```python
from build123d import *

# Parameters (mm, degrees)
BASE_FLANGE1_DEPTH  = 50.8
SKETCH3_R           = 2.7051
TAB1_DEPTH          = 6.35
SKETCH3_2_R         = 2.7051
CUT_EXTRUDE1_DEPTH  = 12.7
SKETCH4_R           = 3.5687
CUT_EXTRUDE2_DEPTH  = 12.7
FILLET1_R           = 6.35
UNFOLD1_START       = 6.35
UNFOLD1_OUTLINE_W   = 50.8
UNFOLD1_OUTLINE_H   = 14.961835013
UNFOLD1_DEPTH       = 95.25
UNFOLD1_2_OUTLINE_R = 2.7051
UNFOLD1_2_DEPTH     = 6.35
FOLD1_START         = -1.304798
FOLD1_DEPTH         = 92.466633013
FOLD1_START_2       = -6.35
FOLD1_2_OUTLINE_R   = 2.7051
FOLD1_2_DEPTH       = 0.034797996
FOLD1_START_3       = -12.7
FOLD1_3_OUTLINE_R   = 2.7051
FOLD1_3_DEPTH       = 12.7
FOLD1_4_DEPTH       = 50.8


with BuildPart() as part:
    # Base-Flange1: sheet metal written as solids
    # Sketch1 → Base-Flange1 (new body)
    with BuildSketch(Plane(origin=(0, 0, 0), x_dir=(0, 0, -1), z_dir=(1, 0, 0))):
        with BuildLine():
            Line((0, 101.6), (0, 12.7))
            ThreePointArc((0, 12.7), (3.719743879, 3.719743879), (12.7, 0))
            Line((12.7, 0), (50.8, 0))
            Line((50.8, 0), (50.8, 6.35))
            Line((50.8, 6.35), (12.7, 6.35))
            ThreePointArc((12.7, 6.35), (8.209871939, 8.209871939), (6.35, 12.7))
            Line((6.35, 12.7), (6.35, 101.6))
            Line((6.35, 101.6), (0, 101.6))
        make_face()
    extrude(amount=BASE_FLANGE1_DEPTH)

    # Tab1: sheet metal written as solids
    # Sketch3 → Tab1 (add)
    with BuildSketch(Plane(origin=(0, 0, -6.35), x_dir=(-1, 0, 0), z_dir=(0, 0, -1))):
        with Locations((-34.925, 23.114)):
            Circle(SKETCH3_R)
        with Locations((-34.925, 88.9)):
            Circle(SKETCH3_R)
        with Locations((-15.875, 38.608)):
            Circle(SKETCH3_R)
        with Locations((-15.875, 78.486)):
            Circle(SKETCH3_R)
    extrude(amount=-TAB1_DEPTH)

    # Sketch3<2> → Cut-Extrude1 (cut)
    with BuildSketch(Plane(origin=(0, 0, -6.35), x_dir=(-1, 0, 0), z_dir=(0, 0, -1))):
        with Locations(Location((-34.925, 23.114, 0), (0, 0, 90))):
            Circle(SKETCH3_2_R)
        with Locations(Location((-34.925, 88.9, 0), (0, 0, 90))):
            Circle(SKETCH3_2_R)
        with Locations(Location((-15.875, 38.608, 0), (0, 0, 90))):
            Circle(SKETCH3_2_R)
        with Locations(Location((-15.875, 78.486, 0), (0, 0, 90))):
            Circle(SKETCH3_2_R)
    extrude(amount=-CUT_EXTRUDE1_DEPTH, mode=Mode.SUBTRACT)

    # Sketch4 → Cut-Extrude2 (cut)
    with BuildSketch(Plane(origin=(0, 6.35, 0), x_dir=(-1, 0, 0), z_dir=(0, 1, 0))):
        with Locations(Location((-41.275, -19.05, 0), (0, 0, 90))):
            Circle(SKETCH4_R)
        with Locations(Location((-9.525, -41.275, 0), (0, 0, 90))):
            Circle(SKETCH4_R)
    extrude(amount=-CUT_EXTRUDE2_DEPTH, mode=Mode.SUBTRACT)

    # Fillet1
    fillet1_edges = [part.edges().sort_by_distance(p)[0] for p in [
        (50.8, 101.6, -3.175),
        (0, 101.6, -3.175),
        (50.8, 3.175, -50.8),
        (0, 3.175, -50.8),
    ]]
    fillet(fillet1_edges, radius=FILLET1_R)

    # Unfold1: read off the stored shape, not the designer's step
    # Unfold1 outline → Unfold1 (cut)
    with BuildSketch(Plane(origin=(0, 0, 0), x_dir=(1, 0, 0), z_dir=(0, 1, 0)).offset(UNFOLD1_START)):
        with Locations((25.4, 5.219082494)):
            Rectangle(UNFOLD1_OUTLINE_W, UNFOLD1_OUTLINE_H)
    extrude(amount=UNFOLD1_DEPTH, mode=Mode.SUBTRACT)

    # Unfold1 2 outline → Unfold1 2 (add)
    with BuildSketch(Plane(origin=(0, 0, 0), x_dir=(1, 0, 0), z_dir=(0, 1, 0))):
        with BuildLine():
            ThreePointArc((0, -84.811835013), (1.859871939, -89.301963073), (6.35, -91.161835013))
            Line((6.35, -91.161835013), (44.45, -91.161835013))
            ThreePointArc((44.45, -91.161835013), (48.940128061, -89.301963073), (50.8, -84.811835013))
            Line((50.8, -84.811835013), (50.8, 12.7))
            Line((50.8, 12.7), (0, 12.7))
            Line((0, 12.7), (0, -84.811835013))
        make_face()
        with Locations((15.875, -68.047835013)):
            Circle(UNFOLD1_2_OUTLINE_R, mode=Mode.SUBTRACT)
        with Locations((34.925, -78.461835013)):
            Circle(UNFOLD1_2_OUTLINE_R, mode=Mode.SUBTRACT)
        with Locations((15.875, -28.169835013)):
            Circle(UNFOLD1_2_OUTLINE_R, mode=Mode.SUBTRACT)
        with Locations((34.925, -12.675835013)):
            Circle(UNFOLD1_2_OUTLINE_R, mode=Mode.SUBTRACT)
    extrude(amount=UNFOLD1_2_DEPTH)

    # Fold1: read off the stored shape, not the designer's step
    # Fold1 outline → Fold1 (cut)
    with BuildSketch(Plane.XY.offset(FOLD1_START)):
        Polygon((50.8, 0), (50.8, 6.35), (0, 6.35), (0, 9e-09), align=None)
    extrude(amount=FOLD1_DEPTH, mode=Mode.SUBTRACT)

    # Fold1 2 outline → Fold1 2 (add)
    with BuildSketch(Plane.XY.offset(FOLD1_START_2)):
        with BuildLine():
            Line((50.8, 6.35), (50.8, 95.25))
            ThreePointArc((50.8, 95.25), (48.940128061, 99.740128061), (44.45, 101.6))
            Line((44.45, 101.6), (6.35, 101.6))
            ThreePointArc((6.35, 101.6), (1.859871939, 99.740128061), (0, 95.25))
            Line((0, 95.25), (0, 6.35))
            Line((0, 6.35), (50.8, 6.35))
        make_face()
        with Locations((15.875, 38.608)):
            Circle(FOLD1_2_OUTLINE_R, mode=Mode.SUBTRACT)
        with Locations((34.925, 23.114)):
            Circle(FOLD1_2_OUTLINE_R, mode=Mode.SUBTRACT)
        with Locations((15.875, 78.486)):
            Circle(FOLD1_2_OUTLINE_R, mode=Mode.SUBTRACT)
        with Locations((34.925, 88.9)):
            Circle(FOLD1_2_OUTLINE_R, mode=Mode.SUBTRACT)
    extrude(amount=FOLD1_2_DEPTH)

    # Fold1 3 outline → Fold1 3 (add)
    with BuildSketch(Plane.XY.offset(FOLD1_START_3)):
        with BuildLine():
            Line((50.8, 6.35), (50.8, 95.25))
            ThreePointArc((50.8, 95.25), (48.940128061, 99.740128061), (44.45, 101.6))
            Line((44.45, 101.6), (6.35, 101.6))
            ThreePointArc((6.35, 101.6), (1.859871939, 99.740128061), (0, 95.25))
            Line((0, 95.25), (0, 6.35))
            Line((0, 6.35), (50.8, 6.35))
        make_face()
        with Locations((15.875, 38.608)):
            Circle(FOLD1_3_OUTLINE_R, mode=Mode.SUBTRACT)
        with Locations((34.925, 23.114)):
            Circle(FOLD1_3_OUTLINE_R, mode=Mode.SUBTRACT)
        with Locations((15.875, 78.486)):
            Circle(FOLD1_3_OUTLINE_R, mode=Mode.SUBTRACT)
        with Locations((34.925, 88.9)):
            Circle(FOLD1_3_OUTLINE_R, mode=Mode.SUBTRACT)
    extrude(amount=FOLD1_3_DEPTH)

    # Fold1 4 outline → Fold1 4 (cut)
    with BuildSketch(Plane.YZ):
        with BuildLine():
            ThreePointArc((9e-09, -12.7), (3.719743885, -3.719743885), (12.7, -9e-09))
            Line((12.7, -9e-09), (6.35, 0))
            Line((6.35, 0), (6.35, -1.304798))
            Line((6.35, -1.304798), (0, -1.304798))
            Line((0, -1.304798), (9e-09, -12.7))
        make_face()
        with BuildLine():
            Line((101.6, -6.35), (12.7, -6.350000009))
            ThreePointArc((12.7, -6.350000009), (8.209871946, -8.209871946), (6.350000009, -12.7))
            Line((6.350000009, -12.7), (101.6, -12.7))
            Line((101.6, -12.7), (101.6, -6.35))
        make_face()
    extrude(amount=FOLD1_4_DEPTH, mode=Mode.SUBTRACT)


solid = part.part
```
Geometry check sheet. Reference: the model listing, model coordinates, mm. Coordinates: 2 decimals unless noted, no trailing zeros. Loops run counter-clockwise (first coordinate to the right, second up) from the corner with the lowest first, then second, coordinate; pieces in that order, holes last. Notation, with made-up numbers: (57, -10.75) -> (72, -10.75) arc R14 ccw to (72, 12.25) -> close; hole circle Ø11 at (46.5, 70.25). An arc over 180 degrees is marked (long way). Put each result on its own line as item: value.
1) Cross-section at D-D on z = -4.5. Record the boundary of the cut face in (x, y) (3 decimals).
Result set:
outline: (0, 3.002) -> (50.8, 3.002) -> (50.8, 95.25) arc R6.35 ccw to (44.45, 101.6) -> (6.35, 101.6) arc R6.35 ccw to (0, 95.25) -> close; hole circle Ø5.41 at (15.875, 38.608); hole circle Ø5.41 at (15.875, 78.486); hole circle Ø5.41 at (34.925, 23.114); hole circle Ø5.41 at (34.925, 88.9)
2) Cross-section at B-B on z = -19.05. Record the boundary of the cut face in (x, y), plus the area to 3 significant figures.
Result set:
outline: (0, 0) -> (37.71, 0) -> (37.71, 6.35) -> (0, 6.35) -> close; (44.84, 0) -> (50.8, 0) -> (50.8, 6.35) -> (44.84, 6.35) -> close
area: 277 mm^2
3) Thickness scan on line 1 (X direction, y = 5, z = -19); line 2 (Z direction, x = 47, y = 56); line 3 (Y direction, x = 19.5, z = -26.5). Record the ranges inside material, lowest first.
Result set:
line 1: x = 0 to 37.71, 44.84 to 50.8
line 2: z = -6.35 to 0
line 3: y = 0 to 6.35
4) Cross-section at C-C on x = 7.5. Record the boundary of the cut face in (y, z), plus the area to 3 significant figures.
Result set:
outline: (0, -50.8) -> (6.35, -50.8) -> (6.35, -44.21) -> (0, -44.21) -> close; (0, -38.34) -> (6.35, -38.34) -> (6.35, -12.7) arc R6.35 cw to (12.7, -6.35) -> (101.6, -6.35) -> (101.6, 0) -> (12.7, 0) arc R12.7 ccw to (0, -12.7) -> close
area: 864 mm^2
5) Release check for a two-part mould opening along Y. For faces 1 (the flat face through (25, 58, -6.35)), 2 (the cylindrical face through (32.223, 23.233, -3.219)), 3 (the flat face through (25, 6.35, -32)) record: released by +Y, released by -Y, zero draft, split by the parting line, or undercut.
Result set:
face 1: zero draft
face 2: undercut
face 3: released by +Y
6) Cross-section at A-A on y = 88.9. Record the boundary of the cut face in (x, z).
Result set:
outline: (0, -6.35) -> (32.22, -6.35) -> (32.22, 0) -> (0, 0) -> close; (37.63, -6.35) -> (50.8, -6.35) -> (50.8, 0) -> (37.63, 0) -> close
7) Gauge pin test, flat ends, axial feed: pin 1 Ø6 at (x, y) = (34.925, 88.9) entering from -Z; pin 2 Ø9.5 at (x, z) = (9.525, -41.275) entering from +Y; pin 3 Ø5.5 at (x, z) = (41.275, -19.05) entering from +Y; pin 4 Ø1.5 at (x, z) = (45.5, -9.5) entering from -Y. Record the tip position at first contact, or that the pin passes through.
Result set:
pin 1: stops at z = -6.35
pin 2: stops at y = 6.35
pin 3: passes through
pin 4: stops at y = 0.24
